Can you work these out from the model? Positions are in its coordinate system, mm. A direction names the side the tool comes from. Give positions to 0.01 mm unless a question says otherwise; leave off trailing zeros. Loops run counter-clockwise (first coordinate to the right, second up) from the corner with the lowest first, then second, coordinate; pieces in that order, holes last. Notation, with made-up numbers: M 41,-34 L 95,-34 A18 ccw 95,-29 Z; hole C 14,19 d7. An arc over 180 degrees is marked long. Answer as a JSON object with one key per item and string values.
```python
from build123d import *
from build123d.topology import SkipClean

# Parameters (mm, degrees)
SKETCH1_R               = 6.5
SKETCH1_R_2             = 1.5
BOSS_EXTRUDE1_DEPTH     = 1
SKETCH2_R               = 4.8
SKETCH2_R_2             = 1.5
BOSS_EXTRUDE2_DEPTH     = 7
SKETCH3_R               = 6.5
SKETCH3_R_2             = 1.5
BOSS_EXTRUDE3_DEPTH     = 1
CROQUIS2_R              = 6.5
CROQUIS2_R_2            = 1.5
SALIENTE_EXTRUIR1_DEPTH = 12
CROQUIS3_R              = 6.5
CROQUIS3_R_2            = 4.8
CORTAR_EXTRUIR2_DEPTH   = 4


with BuildPart() as part:
    # Sketch1 → Boss-Extrude1 (new body)
    with BuildSketch(Plane.XY):
        Circle(SKETCH1_R)
        Circle(SKETCH1_R_2, mode=Mode.SUBTRACT)
    extrude(amount=BOSS_EXTRUDE1_DEPTH)

    # Sketch2 → Boss-Extrude2 (add)
    with BuildSketch(Plane.XY.offset(1)):
        Circle(SKETCH2_R)
        Circle(SKETCH2_R_2, mode=Mode.SUBTRACT)
    extrude(amount=BOSS_EXTRUDE2_DEPTH)

    # Sketch3 → Boss-Extrude3 (add)
    with BuildSketch(Plane.XY.offset(8)):
        Circle(SKETCH3_R)
        Circle(SKETCH3_R_2, mode=Mode.SUBTRACT)
    extrude(amount=BOSS_EXTRUDE3_DEPTH)

    # Croquis2 → Saliente-Extruir1 (add)
    with BuildSketch(Plane.XY.offset(9)):
        Circle(CROQUIS2_R)
        Circle(CROQUIS2_R_2, mode=Mode.SUBTRACT)
    extrude(amount=SALIENTE_EXTRUIR1_DEPTH)

    # Croquis3 → Cortar-Extruir2 (cut)
    with SkipClean():  # the faces are left unmerged after this step: merging them gives an invalid solid
        with BuildSketch(Plane(origin=(0, 0, 8), x_dir=(-1, 0, 0), z_dir=(0, 0, -1))):
            Circle(CROQUIS3_R)
            Circle(CROQUIS3_R_2, mode=Mode.SUBTRACT)
        extrude(amount=-CORTAR_EXTRUIR2_DEPTH, mode=Mode.SUBTRACT)
    add(part.part.scale(1), mode=Mode.REPLACE)  # the faces are merged on a copy


solid = part.part
```
1) Will these pins go through, and if not, where does the flat tip stop? pin 1 Ø1 at (y, z) = (-3.5, 11) entering from +X; pin 2 Ø5 at (x, y) = (0.5, -1) entering from -Z; pin 3 Ø1.8 at (x, y) = (0, 0) entering from -Z; pin 4 Ø1 at (x, z) = (2.5, 14) entering from -Y.
Answer list:
{"pin 1": "x = 3.75", "pin 2": "z = 0", "pin 3": "through", "pin 4": "y = -6.18"}
2) If we mould it in two halves opening along Z, with no side actions, what happens to faces 1 (the flat face through (1, -5, 12)), 2 (the cylindrical face through (-1.5, 0.07, 10.35)), 3 (the flat face through (0, 2, 21))? For each: +Z half, -Z half, draft (parallel to the pull), parting line (faces both ways), or undercut.
Answer list:
{"face 1": "undercut", "face 2": "draft", "face 3": "+Z half"}
3) Suppose I cut it at A-A, the plane x = 0. Write out the boundary of the cut face in (y, z), and give its area (3 significant figures).
Answer list:
{"outline": "M -6.5,0 L -1.5,0 L -1.5,21 L -6.5,21 L -6.5,12 L -4.8,12 L -4.8,1 L -6.5,1 Z; M 1.5,0 L 6.5,0 L 6.5,1 L 4.8,1 L 4.8,12 L 6.5,12 L 6.5,21 L 1.5,21 Z", "area": "173 mm^2"}
4) Suppose I cut it at C-C, the plane z = 18.5. Write out the boundary of the cut face in (x, y), and give its area (3 significant figures).
Answer list:
{"outline": "C 0,0 d13; hole C 0,0 d3", "area": "126 mm^2"}
5) For faces 4 (the flat face through (-1, -5, 1)), 5 (the cylindrical face through (-5.158, -3.955, 0.493)), which set-ups out of +Z, -Z, +X, -X, +Y, -Y let a thin tool reach every point of the face, with its end or its side?
Answer list:
{"face 4": "none", "face 5": "+Z, -Z"}
6) Suppose I cut it at D-D, the plane y = -5.5. Write out the boundary of the cut face in (x, z), and give its area (3 significant figures).
Answer list:
{"outline": "M -3.46,0 L 3.46,0 L 3.46,1 L -3.46,1 Z; M -3.46,12 L 3.46,12 L 3.46,21 L -3.46,21 Z", "area": "69.3 mm^2"}
7) Please list where these lines run through material, in increasing order: line 1 along Z through (x, y) = (-0.75, -6); line 2 along Y through (x, z) = (0, 9.75); line 3 along Y through (x, z) = (0, 17.25). Write a range as from..to.
Answer list:
{"line 1": "0..1, 12..21", "line 2": "-4.8..-1.5, 1.5..4.8", "line 3": "-6.5..-1.5, 1.5..6.5"}
